The listing builds one solid part. Answer for the finished solid, in the listing's coordinates (mm). Round coordinates to 2 decimals unless told otherwise and drop trailing zeros. Order: outer loops, then holes, each group sorted by start corner. A loop starts at its lowest first (then second) coordinate and runs counter-clockwise, first axis right, second up. Notation, with made-up numbers: (46.25, 79.25) -> (84.25, 79.25) arc R30 ccw to (84.25, 118.25) -> close; hole circle Ø8 at (11, 42). An arc over 180 degrees is marked (long way). Return JSON: item names as keys, results as strings. Group by question number.
(1) Consider line 1 (Y direction, x = 1.75, z = -2.5); line 2 (X direction, y = 144.75, z = 0) (3 decimals); line 3 (X direction, y = 5, z = 0) (3 decimals). Determine where each line is inside the solid, lowest interval first. Write a range as [from, to].
(2) Each of these flat-tipped pins is pushed along its axis until it touches: pin 1 (1 mm diameter, centred on x = -1, y = 56.5, fed in from +Z); pin 2 (2 mm diameter, centred on x = 0, z = 0, fed in from +Y); pin 3 (2.5 mm diameter, centred on x = 0, z = 0, fed in from +Y). Where does it stop, or does it pass through?
(3) The part is cut by section A-A (y = 132). Determine the outline of the cut face in (x, z) (3 decimals), plus the area to 3 significant figures.
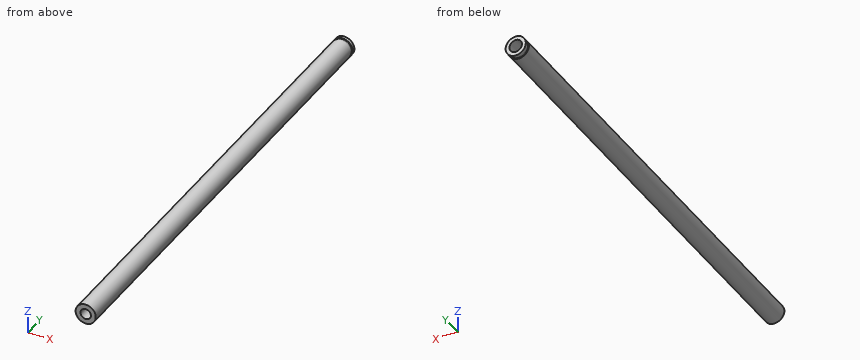
Autodesk Inventor part; units mm, degrees
ref_plane "YZ Plane" through (0, 0, 0) normal (1, 0, 0) x (0, 1, 0)
ref_plane "XZ Plane" through (0, 0, 0) normal (0, 1, 0) x (-1, 0, 0)
ref_plane "XY Plane" through (0, 0, 0) normal (0, 0, 1) x (1, 0, 0)
sketch "Sketch1" plane through (0, 0, 0) normal (0, 0, 1) x (1, 0, 0)
  line L0 (0, 0) -> (0, 149.606)
  line L1 (0, 149.606) -> (3.175, 149.606)
  line L2 (3.175, 149.606) -> (3.175, 148.59)
  line L3 (3.175, 148.59) -> (2.921, 148.59)
  line L4 (2.921, 148.59) -> (2.921, 147.828)
  line L5 (2.921, 147.828) -> (3.175, 147.828)
  line L6 (3.175, 147.828) -> (3.175, 0)
  line L7 (3.175, 0) -> (0, 0)
  dimension "d0" = 3.175
  dimension "d1" = 149.606
  dimension "d2" = 0.762
  dimension "d3" = 0.254
  dimension "d4" = 1.016
revolve "Revolution1" add sketch "Sketch1" angle 360 about axis through (0, 0, 0) along (0, 1, 0)
sketch "Sketch2" plane through (0, 149.606, 0) normal (0, 1, 0) x (1, 0, 0)
  point P0 (0, 0)
  point P1 (0, 0)
hole "Hole1" at (0, 149.606, 0) direction (0, -1, 0) diameter 3.9624 depth 10.16 tip angle 118
sketch "Sketch3" plane through (0, 0, 0) normal (0, -1, 0) x (1, 0, 0)
  point P0 (0, 0)
  point P1 (0, 0)
hole "Hole2" at (0, 0, 0) direction (0, 1, 0) diameter 3.302 depth 10.16 tip angle 118
properties part number "Fixture_Weight_Shaft-02" material "Stainless Steel"
Answer below:
{
 "1": {"line 1": "y = [0, 147.83], [148.59, 149.61]", "line 2": "x = [-3.175, -1.981], [1.981, 3.175]", "line 3": "x = [-3.175, -1.651], [1.651, 3.175]"},
 "2": {"pin 1": "stops at z = 3.14", "pin 2": "stops at y = 138.86", "pin 3": "stops at y = 139.01"},
 "3": {"outline": "circle Ø6.35 at (0, 0)", "area": "31.7 mm²"}
}
